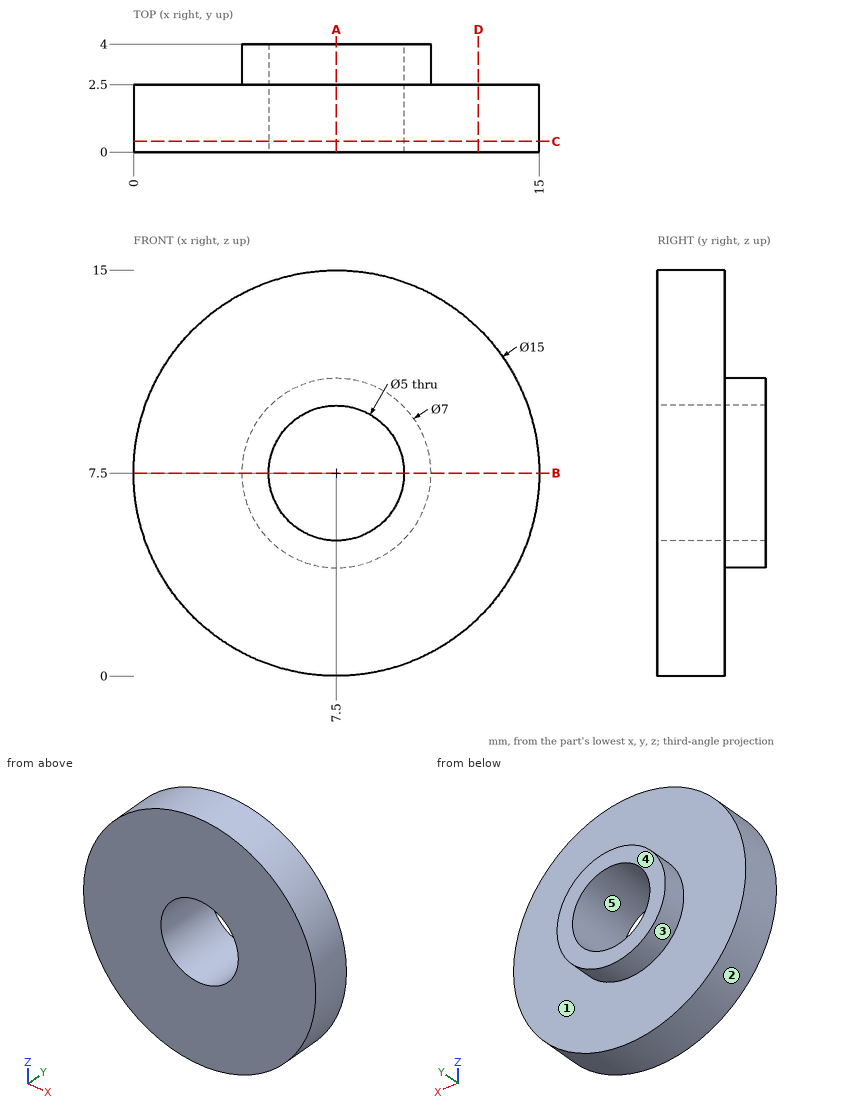
Check sheet for the drawn part. Datum: minimum x, y, z corner. Units: mm. A direction names the side the tool comes from. Round coordinates to 2 decimals unless told otherwise and drop trailing zeros. Write each loop counter-clockwise with the first axis right and the second up, starting at its lowest first coordinate (ties: lowest second). Pieces come first, ordered by that corner, then holes. Notation, with made-up numbers: (71, 54.25) -> (124, 54.25) arc R3 cw to (124, 59.25) -> close; hole circle Ø7 at (-11, 0). An arc over 180 degrees is marked (long way). One line per item, written item: value. Start each with the question number.
(1) Draft check along X on the marked faces 3, 4 and 5. Enter one of: +X half, -X half, draft (parallel to the pull), parting line (faces both ways), or undercut.
(2) Scan lines: line 1 (X direction, y = 2.15, z = 7.5); line 2 (Y direction, x = 5.5, z = 2). Record each from-to range of solid material in increasing order. Write a range as [from, to].
(3) Cross-section at B-B, the plane z = 7.5. Record the cut outline in (x, y), and give its area (3 significant figures).
(4) Cross-section at C-C, the plane y = 0.4. Record the cut outline in (x, z).
(5) Go/stop test with a flat-tipped pin: pin 1 Ø1.5 at (y, z) = (3, 2) entering from +X. Record where the tip stops, or that it passes through.
(6) Cross-section at A-A, the plane x = 7.5. Record the cut outline in (y, z).
(7) Cross-section at D-D, the plane x = 12.75. Record the cut outline in (y, z), and give its area (3 significant figures).
(8) Access from +Z, -Z, +X, -X, +Y, -Y to the whole of each face (thin tool, end or side, straight path). Record for the marked faces 1 and 2.
Answer:
1. face 3: parting line
1. face 4: draft
1. face 5: undercut
2. line 1: [0, 5], [10, 15]
2. line 2: [0, 2.5]
3. outline: (0, 0) -> (5, 0) -> (5, 4) -> (4, 4) -> (4, 2.5) -> (0, 2.5) -> close; (10, 0) -> (15, 0) -> (15, 2.5) -> (11, 2.5) -> (11, 4) -> (10, 4) -> close
3. area: 28.0 mm²
4. outline: circle Ø15 at (7.5, 7.5); hole circle Ø5 at (7.5, 7.5)
5. pin 1: x = 13.14
6. outline: (0, 0) -> (2.5, 0) -> (2.5, 4) -> (4, 4) -> (4, 5) -> (0, 5) -> close; (0, 10) -> (4, 10) -> (4, 11) -> (2.5, 11) -> (2.5, 15) -> (0, 15) -> close
7. outline: (0, 2.14) -> (2.5, 2.14) -> (2.5, 12.86) -> (0, 12.86) -> close
7. area: 26.8 mm²
8. face 1: +Y
8. face 2: +Y, -Y
